Work out the finished part from the listing and answer in its coordinate system (mm). A direction names the side the tool comes from. Round coordinates to 2 decimals unless told otherwise and drop trailing zeros. Loops run counter-clockwise (first coordinate to the right, second up) from the corner with the lowest first, then second, coordinate; pieces in that order, holes last. Notation, with made-up numbers: (27.5, 54.25) - (78.5, 54.25) arc R31 ccw to (78.5, 84.25) - close; hole circle Ø1 at (82.25, 62.5). An arc over 180 degrees is marked (long way). Answer as CSV lines item,"result". Start each with the question number.
Q1. For faces 1 (the face through (-464.844, -1, -3)), 2 (the face through (-451, 0, -41)), 3 (the face through (-411.844, -1, -60)), 4 (the face through (-507.413, -1.479, -24.663)), 5 (the face through (-429, -1, -30.36)), determine the directions among +Z, -Z, +X, -X, +Y, -Y from which every point of the face is accessible in a straight line to the end or side of a thin tool.
Q2. Section A-A on x = -461 is taken. Write down the section's boundary in (y, z), then the cut area to 3 significant figures.
Q3. Section D-D on x = -526 is taken. Write down the section's boundary in (y, z).
Q4. Section B-B on y = -1.1 is taken. Count the separate pieces of the cut face and the enclosed holes in it, then the cut area to 3 significant figures.
Q5. Straight lines are drawn through the part: L1, parallel to Z at x = -508.5, y = -2.65 (3 decimals); L2, parallel to X at y = -1.2, z = -1; L3, parallel to X at y = -0.6, z = -38. For each, find the intervals that lie inside material, in ascending order. Write a range as [from, to].
Q6. Section C-C on z = -85 is taken. Write down the section's boundary in (x, y).
Q7. The mould has two halves that part along X. Classify faces 6 (the face through (-464.844, -1, -35)), 7 (the face through (-533.313, -1.479, -33.144)), 8 (the face through (-451, -3, -41)): +X half, -X half, draft (parallel to the pull), parting line (faces both ways), or undercut.
Q8. Each of these flat-tipped pins is pushed along its axis until it touches: pin 1 Ø17.5 at (x, z) = (-486.84, -25.36) entering from +Y; pin 2 Ø1.5 at (x, y) = (-438.5, -2) entering from -Z; pin 3 Ø1.5 at (x, y) = (-483, -2) entering from +Z; pin 4 Ø1 at (x, y) = (-490.5, -0.5) entering from -Z. Where does it stop, or does it pass through?
```python
from build123d import *

# Parameters (mm, degrees)
ESQUISSE3_R        = 1.5
ESQUISSE3_R_2      = 11
ESQUISSE3_R_3      = 1.7
BOSS_EXTRU_3_DEPTH = 3


with BuildPart() as part:
    # Esquisse3 → Boss.-Extru.3 (new body)
    with BuildSketch(Plane.XZ):
        with BuildLine():
            Line((-464.844143116, -40.359876935), (-411.844143116, -40.359876935))
            Line((-411.844143116, -40.359876935), (-411.844143116, -80.359876935))
            Line((-411.844143116, -80.359876935), (-421.785994494, -113.91817831))
            Line((-421.785994494, -113.91817831), (-501.785994494, -90.217690572))
            Line((-501.785994494, -90.217690572), (-491.844143116, -56.659389197))
            Line((-491.844143116, -56.659389197), (-534.975651854, -43.881416773))
            ThreePointArc((-534.975651854, -43.881416773), (-542.943725497, -33.306292776), (-535.160059098, -22.594711075))
            Line((-535.160059098, -22.594711075), (-496.344143116, -10.359876935))
            Line((-496.344143116, -10.359876935), (-464.844143116, -10.359876935))
            Line((-464.844143116, -10.359876935), (-464.844143116, 4.640123065))
            Line((-464.844143116, 4.640123065), (-394.844143116, 4.640123065))
            Line((-394.844143116, 4.640123065), (-394.844143116, -30.359876935))
            Line((-394.844143116, -30.359876935), (-464.844143116, -30.359876935))
            Line((-464.844143116, -30.359876935), (-464.844143116, -40.359876935))
        make_face()
        with Locations((-531.814143116, -33.209876935)):
            Circle(ESQUISSE3_R, mode=Mode.SUBTRACT)
        with Locations((-508.844143116, -35.113476935)):
            Circle(ESQUISSE3_R, mode=Mode.SUBTRACT)
        with Locations((-508.844143116, -25.113476935)):
            Circle(ESQUISSE3_R, mode=Mode.SUBTRACT)
        with Locations((-486.844143116, -25.359876935)):
            Circle(ESQUISSE3_R_2, mode=Mode.SUBTRACT)
        with Locations((-473.844143116, -25.359876935)):
            Circle(ESQUISSE3_R_3, mode=Mode.SUBTRACT)
        with Locations((-493.344143116, -36.618207185)):
            Circle(ESQUISSE3_R_3, mode=Mode.SUBTRACT)
        with Locations((-493.344143116, -14.101546686)):
            Circle(ESQUISSE3_R_3, mode=Mode.SUBTRACT)
        with Locations((-420.455543116, -55.359876935)):
            Circle(ESQUISSE3_R, mode=Mode.SUBTRACT)
        with Locations((-430.455543116, -55.359876935)):
            Circle(ESQUISSE3_R, mode=Mode.SUBTRACT)
    extrude(amount=BOSS_EXTRU_3_DEPTH)


solid = part.part
```
Findings:
1,face 1,"+Z, -X, +Y, -Y"
1,face 2,"+Z, -Z, +X, -X, +Y"
1,face 3,"-Z, +X, +Y, -Y"
1,face 4,"+Y, -Y"
1,face 5,"+X, +Y, -Y"
2,outline,"(-3, -102.3) - (0, -102.3) - (0, -40.36) - (-3, -40.36) - close; (-3, -30.36) - (0, -30.36) - (0, 4.64) - (-3, 4.64) - close"
2,area,"291 mm^2"
3,outline,"(-3, -46.54) - (0, -46.54) - (0, -19.71) - (-3, -19.71) - close"
4,separate pieces,"1"
4,enclosed holes,"9"
4,area,"9,600 mm^2"
5,L1,"z = [-51.725, -36.573], [-33.653, -26.573], [-23.653, -14.191]"
5,L2,"x = [-464.84, -394.84]"
5,L3,"x = [-541.86, -494.33], [-492.35, -464.84]"
6,outline,"(-500.24, -3) - (-413.22, -3) - (-413.22, 0) - (-500.24, 0) - close"
7,face 6,"+X half"
7,face 7,"undercut"
7,face 8,"draft"
8,pin 1,"passes through"
8,pin 2,"stops at z = -109.19"
8,pin 3,"stops at z = -10.36"
8,pin 4,"stops at z = -93.71"
